```python
from build123d import *

# Parameters (mm, degrees)
F1_DEPTH = 6.35
F2_DEPTH = 6.35
F3_W     = 41.3920721039
F3_H     = 19.1692784429
F4_DEPTH = 25.4
F5_DEPTH = 76.2
F6_W     = 87.5323042274
F6_H     = 20.6641275436
F7_DEPTH = 1270
F8_DEPTH = 127


with BuildPart() as f1:
    # F0 (on Front) → F1 (new body)
    with BuildSketch(Plane.XZ):
        Polygon((13.9693478122, -26.9105285406), (0, -26.9105285406), (-13.9777120203, -26.9105285406), (-23.9575356245, -25.0166002661), (-31.3873849809, -16.4197664708), (-35.2805815637, -23.4119985253), (-36.7282442749, -30.4229743779), (-35.2805815637, -37.568423897), (-26.4761578292, -36.0731184483), (26.4421477914, -36.0731184483), (35.2569408715, -37.568423897), (36.7377512157, -30.4229743779), (35.2569408715, -23.4119985253), (31.3880257308, -16.4197664708), (23.9525288343, -25.0166002661), align=None)
    extrude(amount=F1_DEPTH)

    # F2 (add): a face of the model
    f2_faces = [f1.faces().sort_by_distance(p)[0] for p in [
        (-0.0050105125, 0, -30.0017701646),
    ]]
    extrude(f2_faces, amount=F2_DEPTH)

    # F6 (on face) → F7 (cut)
    with BuildSketch(Plane(origin=(0, 0, -76.2), x_dir=(1, 0, 0), z_dir=(0, 0, -1))):
        with Locations((-0.8414760232, -1.1486634612)):
            Rectangle(F6_W, F6_H)
        Polygon((0, 3.335296642), (36.7744714022, 0), (0, -3.3350162109), (-36.7713794112, 0), align=None, mode=Mode.SUBTRACT)
    extrude(amount=-F7_DEPTH, mode=Mode.SUBTRACT)


with BuildPart() as f4:
    # F3 (on Top) → F4 (new body)
    with BuildSketch(Plane.XY):
        with Locations((5.1154219545, -48.7104393542)):
            Rectangle(F3_W, F3_H)
    extrude(amount=F4_DEPTH)

    # F5 (add): a face of the model
    f5_faces = [f4.faces().sort_by_distance(p)[0] for p in [
        (5.1154219545, -48.7104393542, 0),
    ]]
    extrude(f5_faces, amount=F5_DEPTH)

    # F8 (cut): a face of the model
    f8_faces = [f4.faces().sort_by_distance(p)[0] for p in [
        (5.1154219545, -48.7104393542, -76.2),
    ]]
    extrude(f8_faces, amount=-F8_DEPTH, mode=Mode.SUBTRACT)


solid = f1.part
```
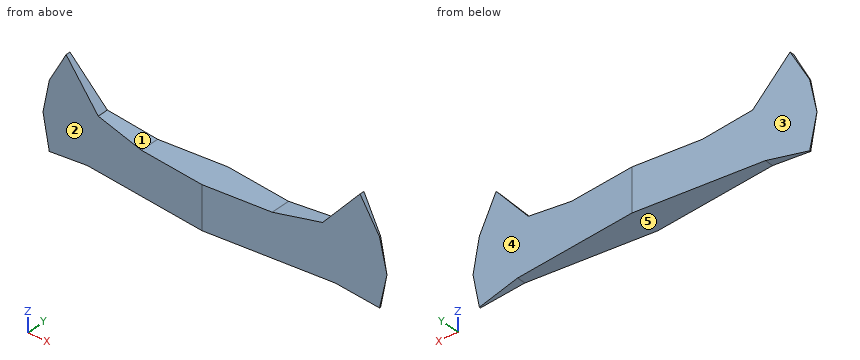
Input: part model. Units: mm. Frame: model coordinates. Face numbers are marked on the shaded views. A direction names the side the tool comes from. Give positions to 0.01 mm unless a question says otherwise; leave off trailing zeros. Loops run counter-clockwise (first coordinate to the right, second up) from the corner with the lowest first, then second, coordinate; pieces in that order, holes last.
1) Mould query, pull axis X, two halves, no side actions, for the marked faces 3, 4 and 5. Classes: released by +X, released by -X, zero draft, split by the parting line, or undercut.
A:
face 3: released by -X
face 4: released by +X
face 5: undercut
2) Section query C-C on z = -32.75. Return the cut outline in (x, y), and give its area (3 significant figures).
A:
outline: (-36.26, -0.05) - (0, -3.34) - (36.26, -0.05) - (36.26, 0.05) - (0, 3.34) - (-36.26, 0.05) - close
area: 245 mm2
3) Section query A-A on z = -28.5. Return the cut outline in (x, y), and give its area (3 significant figures).
A:
outline: (-36.33, -0.04) - (0, -3.34) - (36.33, -0.04) - (36.33, 0.04) - (0, 3.34) - (-36.33, 0.04) - close
area: 245 mm2
4) Line query: L1, parallel to Z at x = -11, y = 1.75; L2, parallel to Y at x = 33, z = -24.5; L3, parallel to Y at x = 10.5, z = -33.25. Output: solid intervals per line, ascending.
A:
L1: z = -36.07 to -26.91
L2: y = -0.34 to 0.34
L3: y = -2.38 to 2.38
5) Section query D-D on x = -30.5. Return the cut outline in (y, z), and give its area (3 significant figures).
A:
outline: (-0.57, -36.76) - (0.57, -36.76) - (0.57, -17.45) - (-0.57, -17.45) - close
area: 22.0 mm2
6) Section query B-B on x = 1. Return the cut outline in (y, z).
A:
outline: (-3.24, -36.07) - (3.24, -36.07) - (3.24, -26.91) - (-3.24, -26.91) - close
7) Reachability of the marked faces 1 and 2 from +Z, -Z, +X, -X, +Y, -Y: full face, straight path, thin tool, end or side. Return the list, or none.
A:
face 1: +Z, +Y, -Y
face 2: +Z, -Z, -X, -Y
8) Contact query for flat-ended pins moving along their axis: pin 1 (8 mm diameter, centred on x = 4.5, z = -27.5, fed in from -Y); pin 2 (1.5 mm diameter, centred on x = -6.5, y = -1, fed in from -Z); pin 3 (4 mm diameter, centred on x = -4.5, z = -25, fed in from -Y). Output: stop coordinate, or through.
A:
pin 1: stops at y = -3.29
pin 2: stops at z = -36.07
pin 3: stops at y = -2.98
